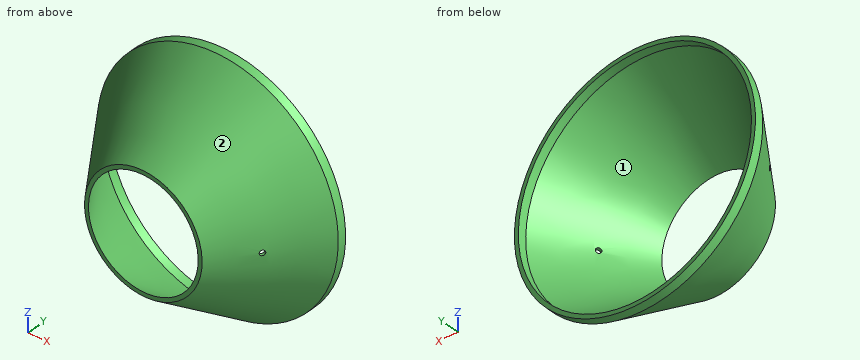
from build123d import *

# Parameters (mm, degrees)
SKETCH36_R          = 0.6
SIDE_HOLES_DEPTH    = 2
CIRPATTERN2_COUNT   = 2
SKETCH37_R          = 27.75
SKETCH37_R_2        = 26.834419058
BOSS_EXTRUDE1_DEPTH = 2


with BuildPart() as part:
    # Sketch35 → Revolve1 (revolve)
    with BuildSketch(Plane.XY, mode=Mode.PRIVATE) as revolve1_sk:
        Polygon((12.63, 0), (13.545580942, 0), (27.75, 20.286012765), (26.834419058, 20.286012765), align=None)
    revolve(revolve1_sk.sketch.rotate(Axis((0, 20.286012765, 0), (0, -1, 0)), 90), axis=Axis((0, 20.286012765, 0), (0, -1, 0)))

    # Sketch36 → side-holes (cut, symmetric)
    with BuildSketch(Plane(origin=(8.474857205, -5.9341589, 0), x_dir=(0, 0, 1), z_dir=(-0.8191520442889934, 0.5735764363510439, 0))):
        with Locations(Location((0, 18.744270391, 0), (0, 0, 235.340174101))):
            Circle(SKETCH36_R)
    side_holes = extrude(amount=SIDE_HOLES_DEPTH, both=True, mode=Mode.SUBTRACT)

    # CirPattern2: side-holes ×2 about axis
    cirpattern2_axis = Axis((0, 0, 0), (0, 1, 0))
    for i in range(1, CIRPATTERN2_COUNT):
        add(side_holes.rotate(cirpattern2_axis, i * 360 / CIRPATTERN2_COUNT), mode=Mode.SUBTRACT)

    # Sketch37 → Boss-Extrude1 (add)
    with BuildSketch(Plane(origin=(0, 20.286012765, 0), x_dir=(1, 0, 0), z_dir=(0, 1, 0))):
        with Locations(Location((0, 0, 0), (0, 0, 270))):
            Circle(SKETCH37_R)
        with Locations(Location((0, 0, 0), (0, 0, 270))):
            Circle(SKETCH37_R_2, mode=Mode.SUBTRACT)
    extrude(amount=BOSS_EXTRUDE1_DEPTH)


solid = part.part
Model file for the job. Use its own axes, mm. Face numbers are marked on the shaded views. Round coordinates to 2 decimals unless told otherwise and drop trailing zeros. Loops run counter-clockwise (first coordinate to the right, second up) from the corner with the lowest first, then second, coordinate; pieces in that order, holes last.
1. Mould opens along X. For the marked faces 1 and 2 say: +X half, -X half, draft (parallel to the pull), parting line (faces both ways), or undercut.
Check values:
face 1: undercut
face 2: parting line
2. Drop flat-ended pins along their axis: P1, Ø8, axis at x = 20, z = -6.5, coming from the +Y side; P2, Ø1, axis at x = 21.5, y = 19, coming from the -Z side; P3, Ø10, axis at x = 14.5, z = 7.5, coming from the -Y side; P4, Ø4, axis at y = 2, z = 1, coming from the +X side. Give the stop position or say it passes through.
Check values:
P1: stops at y = 17.71
P2: stops at z = -16.94
P3: stops at y = 0
P4: stops at x = 16.32
3. Band-saw the part on C-C, the plane y = 7. List the corners of the cut face in (x, z), and give its area (3 significant figures).
Check values:
outline: circle Ø36.89 at (0, 0); hole circle Ø35.06 at (0, 0)
area: 103 mm2
4. Wall check: probe 1 along Z at (x, y) = (0, 21); probe 2 along Z at (x, y) = (17, 19.5). Give the ranges that are in metal, low to high.
Check values:
probe 1: z = -27.75 to -26.83, 26.83 to 27.75
probe 2: z = -21.23 to -20.05, 20.05 to 21.23
5. Band-saw the part on B-B, the plane y = 12. List the corners of the cut face in (x, z).
Check values:
outline: circle Ø43.9 at (0, 0); hole circle Ø42.06 at (0, 0)
